from build123d import *

# Parameters (mm, degrees)
F1_DEPTH = 25
F3_START = -0.65
F2_R     = 4.3
F3_DEPTH = 2.15
F6_DEPTH = 23
F7_R     = 33.55183595
F8_DEPTH = 2


with BuildPart() as f1:
    # F0 (on Top) → F1 (new body)
    with BuildSketch(Plane.XY):
        with BuildLine():
            ThreePointArc((7.6794919243, -4), (19.8038475773, 3), (19.8038475773, 17))
            Line((19.8038475773, 17), (12.124355653, 30.3012701892))
            ThreePointArc((12.124355653, 30.3012701892), (0, 37.3012701892), (-12.124355653, 30.3012701892))
            Line((-12.124355653, 30.3012701892), (-19.8038475773, 17))
            ThreePointArc((-19.8038475773, 17), (-19.8038475773, 3), (-7.6794919243, -4))
            Line((-7.6794919243, -4), (0, -4))
            Line((0, -4), (7.6794919243, -4))
        make_face()
        with BuildLine():
            Line((7.6794919243, 0), (0, 0))
            Line((0, 0), (-7.6794919243, 0))
            ThreePointArc((-7.6794919243, 0), (-16.3397459622, 5), (-16.3397459622, 15))
            Line((-16.3397459622, 15), (-8.6602540378, 28.3012701892))
            ThreePointArc((-8.6602540378, 28.3012701892), (0, 33.3012701892), (8.6602540378, 28.3012701892))
            Line((8.6602540378, 28.3012701892), (16.3397459622, 15))
            ThreePointArc((16.3397459622, 15), (16.3397459622, 5), (7.6794919243, 0))
        make_face(mode=Mode.SUBTRACT)
    extrude(amount=F1_DEPTH)

    # F2 (on face) → F3 (cut)
    with BuildSketch(Plane(origin=(-22.2141016151, 12.8253175473, 0), x_dir=(-0.5, -0.8660254038, 0), z_dir=(-0.8660254038, 0.5, 0)).offset(F3_START)):
        with Locations((-12.5, 12.5)):
            Circle(F2_R)
    extrude(amount=-F3_DEPTH, mode=Mode.SUBTRACT)

    # F5 (on face) → F6 (cut)
    with BuildSketch(Plane(origin=(0, 0, 0), x_dir=(1, 0, 0), z_dir=(0, 0, -1))):
        with BuildLine():
            Line((-19.2409310648, -16.675), (-11.5614391405, -29.9762701892))
            ThreePointArc((-11.5614391405, -29.9762701892), (0, -36.6512701892), (11.5614391405, -29.9762701892))
            Line((11.5614391405, -29.9762701892), (19.2409310648, -16.675))
            ThreePointArc((19.2409310648, -16.675), (19.2409310648, -3.325), (7.6794919243, 3.35))
            Line((7.6794919243, 3.35), (-7.6794919243, 3.35))
            ThreePointArc((-7.6794919243, 3.35), (-19.2409310648, -3.325), (-19.2409310648, -16.675))
        make_face()
    extrude(amount=-F6_DEPTH, mode=Mode.SUBTRACT)

    # F7 (on face) → F8 (cut)
    with BuildSketch(Plane(origin=(0, 0, 0), x_dir=(1, 0, 0), z_dir=(0, 0, -1))):
        with Locations((-1.2054177932, -16.7930107564)):
            Circle(F7_R)
    extrude(amount=-F8_DEPTH, mode=Mode.SUBTRACT)


solid = f1.part
Here's how the part is built. I have some questions about the finished solid (model axes, mm). A direction names the side the tool comes from. Coordinates: 2 decimals unless noted, no trailing zeros. Write each loop counter-clockwise with the first axis right and the second up, starting at its lowest first coordinate (ties: lowest second). Pieces come first, ordered by that corner, then holes.
Item 1: I want a section at B-B on x = -5. Write out the boundary of the cut face in (y, z), and give its area (3 significant figures).
Item 2: If we mould it in two halves opening along X, with no side actions, what happens to faces 4 (the cylindrical face through (-19.905, 3.178, 13.339)), 5 (the flat face through (0, -3.35, 12)), 6 (the cylindrical face through (19.7, 2.82, 13.34)), 7 (the flat face through (0, 0, 24))? For each: +X half, -X half, draft (parallel to the pull), parting line (faces both ways), or undercut.
Item 3: If I drill on line 1 (Y direction, x = 0.5, z = 18); line 2 (Z direction, x = -18, y = 9.5); line 3 (Y direction, x = 14.5, z = 6.5), over which ranges is the centre line in solid material (lowest first)?
Item 4: Will these pins go through, and if not, where does the flat tip stop? pin 1 (10 mm diameter, centred on x = 4.5, y = 29.5, fed in from -Z); pin 2 (1.5 mm diameter, centred on y = 24.5, z = 14, fed in from -X); pin 3 (2 mm diameter, centred on x = -1.5, z = 24, fed in from +Y).
Item 5: On a 3-axis mill with a long thin cutter (end or side, diameter ignored), from which of +Z, -Z, +X, -X, +Y, -Y can I reach the whole of each face in a straight line? I mean faces 1 (the flat face through (-11.3, 24.4, 25)), 2 (the flat face through (0, -1, 23)), 3 (the cylindrical face through (-0.1, 33.3, 24)). Say none if no direction works.
Item 6: I want a section at D-D on x = -14.5. Write out the boundary of the cut face in (y, z).
Item 7: I want a section at A-A on y = 11.5. Write out the boundary of the cut face in (x, z), and give its area (3 significant figures).
Findings below:
1. outline: (-4, 2) - (-3.35, 2) - (-3.35, 23) - (0, 23) - (0, 25) - (-4, 25) - close; (31.96, 23) - (35.68, 23) - (35.68, 2) - (36.38, 2) - (36.38, 25) - (31.96, 25) - close
1. area: 45.1 mm2
2. face 4: -X half
2. face 5: undercut
2. face 6: +X half
2. face 7: undercut
3. line 1: y = -4 to -3.35, 36.64 to 37.29
3. line 2: z = 23 to 25
3. line 3: y = -2.23 to -1.48, 24.89 to 26.19
4. pin 1: stops at z = 23
4. pin 2: stops at x = -15.91
4. pin 3: stops at y = 37.29
5. face 1: +Z, +X, -X, +Y, -Y
5. face 2: -Z
5. face 3: +Z, -Z
6. outline: (-2.23, 2) - (-1.48, 2) - (-1.48, 23) - (2.69, 23) - (2.69, 25) - (-2.23, 25) - close; (18.19, 23) - (24.89, 23) - (24.89, 2) - (26.19, 2) - (26.19, 25) - (18.19, 25) - close
7. outline: (-21.6, 2) - (-20.94, 2) - (-20.94, 23) - (-17.57, 23) - (-17.57, 25) - (-21.6, 25) - close; (17.57, 23) - (20.94, 23) - (20.94, 2) - (21.6, 2) - (21.6, 25) - (17.57, 25) - close
7. area: 43.6 mm2
